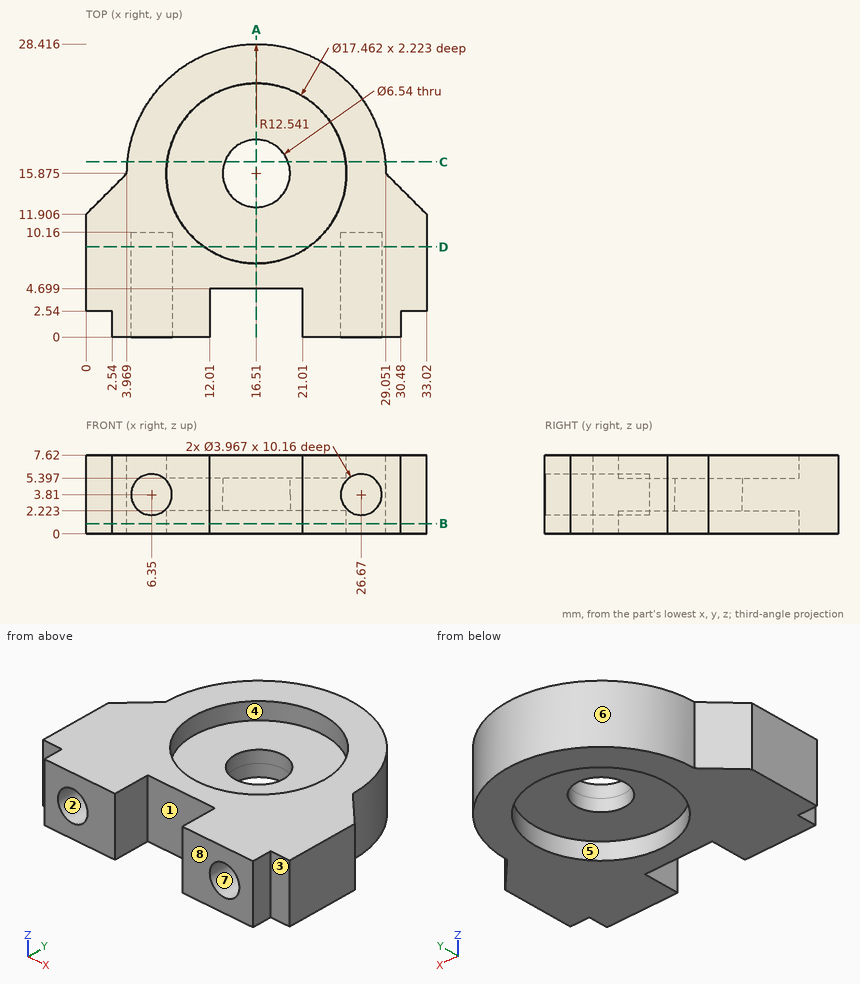
Here's the drawing with two shaded views (mm, measured from the low corner). I have some questions. A direction names the side the tool comes from. Coordinates: 2 decimals unless noted, no trailing zeros. Order: outer loops, then holes, each group sorted by start corner. A loop starts at its lowest first (then second) coordinate and runs counter-clockwise, first axis right, second up. Notation, with made-up numbers: (43, 19) - (66, 19) arc R28 ccw to (66, 37) - close; hole circle Ø11 at (-3.5, 48). An arc over 180 degrees is marked (long way). Answer in a Markdown table with one row per item. Add a question column.
(1) If we mould it in two halves opening along X, with no side actions, what happens to the marked faces 6, 7 and 8? For each: released by +X, released by -X, zero draft, split by the parting line, or undercut.
(2) Will these pins go through, and if not, where does the flat tip stop? pin 1 (3 mm diameter, centred on x = 16.5, y = 16, fed in from -Z); pin 2 (2 mm diameter, centred on x = 20.5, y = 21, fed in from +Z); pin 3 (0.8 mm diameter, centred on y = 2, z = 4.5, fed in from +X); pin 4 (3 mm diameter, centred on x = 6.5, z = 4, fed in from -Y).
(3) If we section it at C-C, the plane y = 17: Please give me the cut outline in (x, z).
(4) I need wall thicknesses on L1, parallel to X at y = 5.5, z = 3.81; L2, parallel to Z at x = 26.67, y = 4.5; L3, parallel to Y at x = 16.51, z = 6.3. Which ranges of each line are inside material? Lowest first, please.
(5) If we section it at B-B, the plane z = 1: Please give me the cut outline in (x, y) (1 decimal), then the cut area to 3 significant figures.
(6) If we section it at D-D, the plane y = 8.75: Please give me the cut outline in (x, z).
(7) On a 3-axis mill with a long thin cutter (end or side, diameter ignored), from which of +Z, -Z, +X, -X, +Y, -Y can I reach the whole of each face in a straight line? I mean the marked faces 1, 2, 3, 4 and 5. Say none if no direction works.
(8) If we section it at A-A, the plane x = 16.51: Please give me the cut outline in (y, z) (1 decimal).
Results are:
| question | item | result |
|---|---|---|
| 1 | face 6 | split by the parting line |
| 1 | face 7 | undercut |
| 1 | face 8 | zero draft |
| 2 | pin 1 | passes through |
| 2 | pin 2 | stops at z = 5.4 |
| 2 | pin 3 | stops at x = 30.48 |
| 2 | pin 4 | stops at y = 10.16 |
| 3 | outline | (4.02, 0) - (7.85, 0) - (7.85, 2.22) - (13.44, 2.22) - (13.44, 5.4) - (7.85, 5.4) - (7.85, 7.62) - (4.02, 7.62) - close; (19.58, 2.22) - (25.17, 2.22) - (25.17, 0) - (29, 0) - (29, 7.62) - (25.17, 7.62) - (25.17, 5.4) - (19.58, 5.4) - close |
| 4 | L1 | x = 0 to 4.37, 8.33 to 24.69, 28.65 to 33.02 |
| 4 | L2 | z = 0 to 1.83, 5.79 to 7.62 |
| 4 | L3 | y = 4.7 to 7.14, 24.61 to 28.42 |
| 5 | outline | (0, 2.5) - (2.5, 2.5) - (2.5, 0) - (12, 0) - (12, 4.7) - (21, 4.7) - (21, 0) - (30.5, 0) - (30.5, 2.5) - (33, 2.5) - (33, 11.9) - (29.1, 15.9) arc R12.5 ccw to (4, 15.9) - (0, 11.9) - close; hole circle Ø17.5 at (16.5, 15.9) |
| 5 | area | 461 mm2 |
| 6 | outline | (0, 0) - (11.46, 0) - (11.46, 2.22) - (21.56, 2.22) - (21.56, 0) - (33.02, 0) - (33.02, 7.62) - (21.56, 7.62) - (21.56, 5.4) - (11.46, 5.4) - (11.46, 7.62) - (0, 7.62) - close; hole circle Ø3.97 at (6.35, 3.81); hole circle Ø3.97 at (26.67, 3.81) |
| 7 | face 1 | +Z, -Z, -Y |
| 7 | face 2 | -Y |
| 7 | face 3 | +Z, -Z, +X, -Y |
| 7 | face 4 | +Z |
| 7 | face 5 | -Z |
| 8 | outline | (4.7, 0) - (7.1, 0) - (7.1, 2.2) - (12.6, 2.2) - (12.6, 5.4) - (7.1, 5.4) - (7.1, 7.6) - (4.7, 7.6) - close; (19.1, 2.2) - (24.6, 2.2) - (24.6, 0) - (28.4, 0) - (28.4, 7.6) - (24.6, 7.6) - (24.6, 5.4) - (19.1, 5.4) - close |
